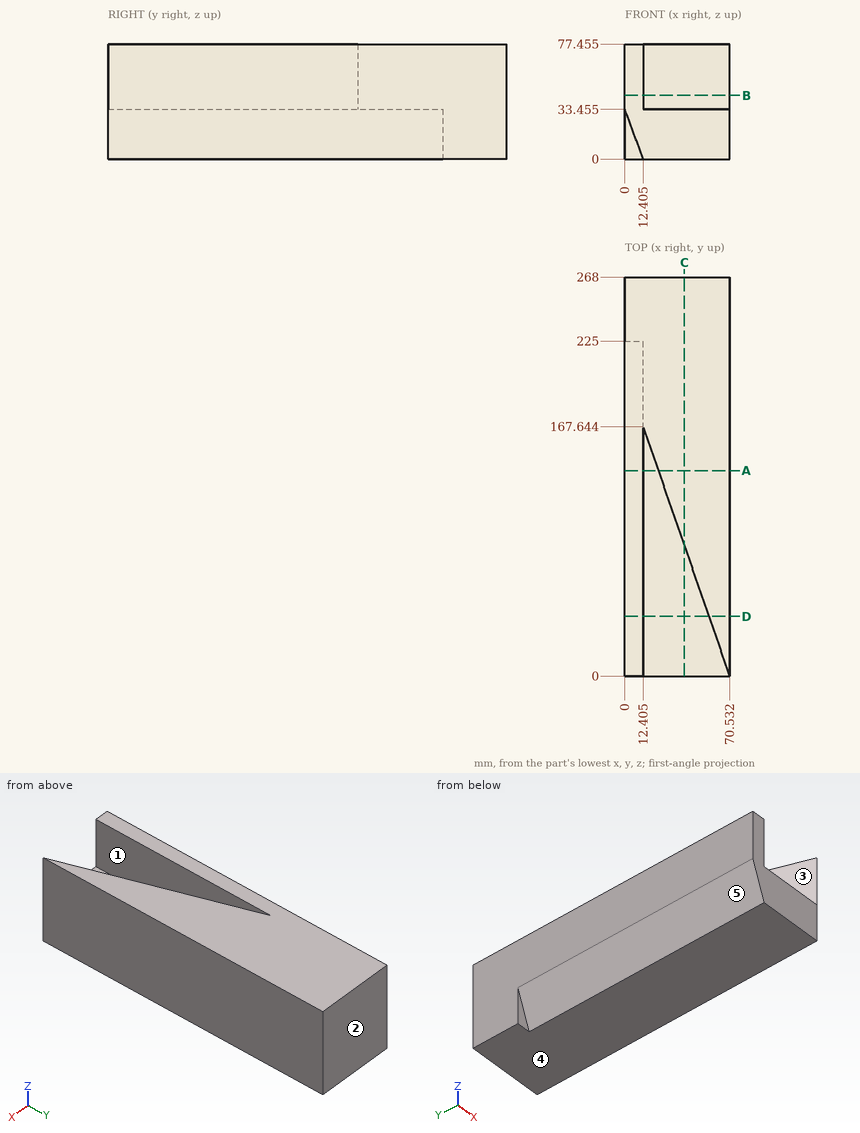
Part print with two shaded views. Sizes in mm from the minimum x, y, z corner. A direction names the side the tool comes from. Round coordinates to 2 decimals unless told otherwise and drop trailing zeros. Order: outer loops, then holes, each group sorted by start corner. A loop starts at its lowest first (then second) coordinate and runs counter-clockwise, first axis right, second up. Notation, with made-up numbers: (61.25, 70) - (84.25, 70) arc R33 ccw to (84.25, 109) - close; hole circle Ø9 at (-16, -32.5). An arc over 180 degrees is marked (long way). Return JSON: item names as keys, results as strings.
(1) Cut at A-A (y = 138). Give the cut face in (x, z) (1 decimal), then the cut area to 3 significant figures.
Answer key:
{"outline": "(0, 33.5) - (12.4, 0) - (70.5, 0) - (70.5, 77.5) - (22.7, 77.5) - (22.7, 33.5) - (12.4, 33.5) - (12.4, 77.5) - (0, 77.5) - close", "area": "4,800 mm^2"}
(2) Cut at C-C (x = 40). Give the cut face in (y, z) (1 decimal).
Answer key:
{"outline": "(0, 0) - (268, 0) - (268, 77.5) - (88.1, 77.5) - (88.1, 33.5) - (0, 33.5) - close"}
(3) Pin check, flat tips, straight feed: pin 1 Ø3.5 at (x, z) = (5.5, 15) entering from -Y; pin 2 Ø5 at (x, y) = (21, 52.5) entering from +Z (1 decimal). Stop position of each tip, or through.
Answer key:
{"pin 1": "stops at y = 0", "pin 2": "stops at z = 33.5"}
(4) Cut at D-D (y = 40). Give the cut face in (x, z) (1 decimal).
Answer key:
{"outline": "(0, 33.5) - (12.4, 0) - (70.5, 0) - (70.5, 77.5) - (56.7, 77.5) - (56.7, 33.5) - (12.4, 33.5) - (12.4, 77.5) - (0, 77.5) - close"}
(5) Cut at B-B (z = 43). Give the cut face in (x, y) (1 decimal).
Answer key:
{"outline": "(0, 0) - (12.4, 0) - (12.4, 167.6) - (70.5, 0) - (70.5, 268) - (0, 268) - close"}
(6) Tool access for the marked faces 1 and 2: list every direction of +Z, -Z, +X, -X, +Y, -Y with a clear straight run to the whole face (end or side of a thin tool).
Answer key:
{"face 1": "+Z, -Y", "face 2": "+Z, -Z, +X, -X, +Y"}
(7) Wall check: probe 1 along Z at (x, y) = (17, 90.5) (1 decimal); probe 2 along X at (y, z) = (108.5, 51) (1 decimal); probe 3 along X at (y, z) = (138, 69) (1 decimal). Give the ranges that are in metal, low to high. Write a range as from..to.
Answer key:
{"probe 1": "z = 0..33.5", "probe 2": "x = 0..12.4, 32.9..70.5", "probe 3": "x = 0..12.4, 22.7..70.5"}
(8) Pull direction X, two halves, no side cores. Call the marked faces 3, 4 and 5: +X half, -X half, draft (parallel to the pull), parting line (faces both ways), or undercut.
Answer key:
{"face 3": "undercut", "face 4": "draft", "face 5": "-X half"}
